Check sheet for the modelled part. Datum: model origin and axes. Units: mm. A direction names the side the tool comes from. Round coordinates to 2 decimals unless told otherwise and drop trailing zeros. Order: outer loops, then holes, each group sorted by start corner. A loop starts at its lowest first (then second) coordinate and runs counter-clockwise, first axis right, second up. Notation, with made-up numbers: (34, 12.25) -> (49, 12.25) arc R22 cw to (49, 27.25) -> close; hole circle Ø10 at (-14.75, -5.75). An arc over 180 degrees is marked (long way). Answer in a Markdown table with one row per item.
from build123d import *

# Parameters (mm, degrees)
SKETCH1_R                                       = 12
SKETCH1_R_2                                     = 1.65
BOSS_EXTRUDE1_DEPTH                             = 15
SKETCH2_R                                       = 20
SKETCH2_R_2                                     = 11.285963192
BOSS_EXTRUDE2_DEPTH                             = 5
SKETCH3_R                                       = 20
BOSS_EXTRUDE3_DEPTH                             = 3
CUT_EXTRUDE2_DEPTH                              = 2.1
SKETCH6_R                                       = 1.65
CUT_EXTRUDE3_DEPTH                              = 24.1
FILLET1_R                                       = 1
SKETCH7_R                                       = 3.5
CUT_EXTRUDE4_DEPTH                              = 5.5
CSK_FOR_M3_FLAT_HEAD_MACHINE_SCREW1_D           = 3.4
CSK_FOR_M3_FLAT_HEAD_MACHINE_SCREW1_CSINK_D     = 6.3
CSK_FOR_M3_FLAT_HEAD_MACHINE_SCREW1_CSINK_ANGLE = 90
CUT_EXTRUDE6_DEPTH                              = 2
CUT_EXTRUDE6_DEPTH_BACK                         = 10


with BuildPart() as part:
    # Sketch1 → Boss-Extrude1 (new body)
    with BuildSketch(Plane(origin=(0, 0, 0), x_dir=(1, 0, 0), z_dir=(0, 1, 0))):
        Circle(SKETCH1_R)
        with Locations((0, 7)):
            Circle(SKETCH1_R_2, mode=Mode.SUBTRACT)
        with Locations((7, 0)):
            Circle(SKETCH1_R_2, mode=Mode.SUBTRACT)
        Circle(SKETCH1_R_2, mode=Mode.SUBTRACT)
        with Locations((0, -7)):
            Circle(SKETCH1_R_2, mode=Mode.SUBTRACT)
        with Locations((-7, 0)):
            Circle(SKETCH1_R_2, mode=Mode.SUBTRACT)
    extrude(amount=BOSS_EXTRUDE1_DEPTH)

    # Sketch2 → Boss-Extrude2 (add)
    with BuildSketch(Plane(origin=(0, 15, 0), x_dir=(1, 0, 0), z_dir=(0, 1, 0))):
        Circle(SKETCH2_R)
        Circle(SKETCH2_R_2, mode=Mode.SUBTRACT)
    extrude(amount=-BOSS_EXTRUDE2_DEPTH)

    # Sketch3 → Boss-Extrude3 (add)
    with BuildSketch(Plane(origin=(0, 15, 0), x_dir=(1, 0, 0), z_dir=(0, 1, 0))):
        Circle(SKETCH3_R)
    extrude(amount=-BOSS_EXTRUDE3_DEPTH)

    # Sketch4 → Cut-Extrude2 (cut)
    with BuildSketch(Plane.XZ.offset(-15)):
        with BuildLine():
            Line((4.949747468, 4.949747468), (1.940261042, 16.98516707))
            ThreePointArc((1.940261042, 16.98516707), (0, 18.5), (-1.940261043, 16.98516707))
            Line((-1.940261043, 16.98516707), (-4.949747468, 4.949747468))
            Line((-4.949747468, 4.949747468), (-16.98516707, 1.940261042))
            ThreePointArc((-16.98516707, 1.940261042), (-18.5, 0), (-16.98516707, -1.940261043))
            Line((-16.98516707, -1.940261043), (-4.949747468, -4.949747468))
            Line((-4.949747468, -4.949747468), (-1.940261042, -16.98516707))
            ThreePointArc((-1.940261042, -16.98516707), (0, -18.5), (1.940261043, -16.98516707))
            Line((1.940261043, -16.98516707), (4.949747468, -4.949747468))
            Line((4.949747468, -4.949747468), (16.98516707, -1.940261042))
            ThreePointArc((16.98516707, -1.940261042), (18.5, 0), (16.98516707, 1.940261043))
            Line((16.98516707, 1.940261043), (4.949747468, 4.949747468))
        make_face()
    extrude(amount=CUT_EXTRUDE2_DEPTH, mode=Mode.SUBTRACT)

    # Sketch6 → Cut-Extrude3 (cut)
    with BuildSketch(Plane.XZ):
        Circle(SKETCH6_R)
    extrude(amount=-CUT_EXTRUDE3_DEPTH, mode=Mode.SUBTRACT)

    # Fillet1
    fillet1_edges = [part.edges().sort_by_distance(p)[0] for p in [
        (4.949747468, 13.95, 4.949747468),
        (-4.949747468, 13.95, 4.949747468),
        (-4.949747468, 13.95, -4.949747468),
        (4.949747468, 13.95, -4.949747468),
    ]]
    fillet(fillet1_edges, radius=FILLET1_R)

    # Sketch7 → Cut-Extrude4 (cut)
    with BuildSketch(Plane.XZ):
        Circle(SKETCH7_R)
    extrude(amount=-CUT_EXTRUDE4_DEPTH, mode=Mode.SUBTRACT)

    # CSK for M3 Flat Head Machine Screw1 (through all)
    with Locations(Plane(origin=(0, 5.5, 0), x_dir=(-1, 0, 0), z_dir=(0, -1, 0))):
        with Locations((0, 0)):
            CounterSinkHole(CSK_FOR_M3_FLAT_HEAD_MACHINE_SCREW1_D / 2, CSK_FOR_M3_FLAT_HEAD_MACHINE_SCREW1_CSINK_D / 2, counter_sink_angle=CSK_FOR_M3_FLAT_HEAD_MACHINE_SCREW1_CSINK_ANGLE)

    # Sketch12 → Cut-Extrude6 (cut, two sides)
    with BuildSketch(Plane.XZ.offset(-12)) as cut_extrude6_sk:
        with BuildLine():
            Line((-2.836233197, 8.522029946), (-2.836233197, 5.477970054))
            ThreePointArc((-2.836233197, 5.477970054), (-2.809438278, 5.377970054), (-2.736233197, 5.304764973))
            Line((-2.736233197, 5.304764973), (-0.1, 3.782735027))
            ThreePointArc((-0.1, 3.782735027), (0, 3.755940108), (0.1, 3.782735027))
            Line((0.1, 3.782735027), (2.736233197, 5.304764973))
            ThreePointArc((2.736233197, 5.304764973), (2.809438278, 5.377970054), (2.836233197, 5.477970054))
            Line((2.836233197, 5.477970054), (2.836233197, 8.522029946))
            ThreePointArc((2.836233197, 8.522029946), (2.809438278, 8.622029946), (2.736233197, 8.695235027))
            Line((2.736233197, 8.695235027), (0.1, 10.217264973))
            ThreePointArc((0.1, 10.217264973), (0, 10.244059892), (-0.1, 10.217264973))
            Line((-0.1, 10.217264973), (-2.736233197, 8.695235027))
            ThreePointArc((-2.736233197, 8.695235027), (-2.809438278, 8.622029946), (-2.836233197, 8.522029946))
        make_face()
        with BuildLine():
            Line((-10.217264973, -0.1), (-8.695235027, -2.736233197))
            ThreePointArc((-8.695235027, -2.736233197), (-8.622029946, -2.809438278), (-8.522029946, -2.836233197))
            Line((-8.522029946, -2.836233197), (-5.477970054, -2.836233197))
            ThreePointArc((-5.477970054, -2.836233197), (-5.377970054, -2.809438278), (-5.304764973, -2.736233197))
            Line((-5.304764973, -2.736233197), (-3.782735027, -0.1))
            ThreePointArc((-3.782735027, -0.1), (-3.755940108, 0), (-3.782735027, 0.1))
            Line((-3.782735027, 0.1), (-5.304764973, 2.736233197))
            ThreePointArc((-5.304764973, 2.736233197), (-5.377970054, 2.809438278), (-5.477970054, 2.836233197))
            Line((-5.477970054, 2.836233197), (-8.522029946, 2.836233197))
            ThreePointArc((-8.522029946, 2.836233197), (-8.622029946, 2.809438278), (-8.695235027, 2.736233197))
            Line((-8.695235027, 2.736233197), (-10.217264973, 0.1))
            ThreePointArc((-10.217264973, 0.1), (-10.244059892, 0), (-10.217264973, -0.1))
        make_face()
        with BuildLine():
            Line((8.522029946, 2.836233197), (5.477970054, 2.836233197))
            ThreePointArc((5.477970054, 2.836233197), (5.377970054, 2.809438278), (5.304764973, 2.736233197))
            Line((5.304764973, 2.736233197), (3.782735027, 0.1))
            ThreePointArc((3.782735027, 0.1), (3.755940108, 0), (3.782735027, -0.1))
            Line((3.782735027, -0.1), (5.304764973, -2.736233197))
            ThreePointArc((5.304764973, -2.736233197), (5.377970054, -2.809438278), (5.477970054, -2.836233197))
            Line((5.477970054, -2.836233197), (8.522029946, -2.836233197))
            ThreePointArc((8.522029946, -2.836233197), (8.622029946, -2.809438278), (8.695235027, -2.736233197))
            Line((8.695235027, -2.736233197), (10.217264973, -0.1))
            ThreePointArc((10.217264973, -0.1), (10.244059892, 0), (10.217264973, 0.1))
            Line((10.217264973, 0.1), (8.695235027, 2.736233197))
            ThreePointArc((8.695235027, 2.736233197), (8.622029946, 2.809438278), (8.522029946, 2.836233197))
        make_face()
        with BuildLine():
            Line((2.836233197, -8.522029946), (2.836233197, -5.477970054))
            ThreePointArc((2.836233197, -5.477970054), (2.809438278, -5.377970054), (2.736233197, -5.304764973))
            Line((2.736233197, -5.304764973), (0.1, -3.782735027))
            ThreePointArc((0.1, -3.782735027), (0, -3.755940108), (-0.1, -3.782735027))
            Line((-0.1, -3.782735027), (-2.736233197, -5.304764973))
            ThreePointArc((-2.736233197, -5.304764973), (-2.809438278, -5.377970054), (-2.836233197, -5.477970054))
            Line((-2.836233197, -5.477970054), (-2.836233197, -8.522029946))
            ThreePointArc((-2.836233197, -8.522029946), (-2.809438278, -8.622029946), (-2.736233197, -8.695235027))
            Line((-2.736233197, -8.695235027), (-0.1, -10.217264973))
            ThreePointArc((-0.1, -10.217264973), (0, -10.244059892), (0.1, -10.217264973))
            Line((0.1, -10.217264973), (2.736233197, -8.695235027))
            ThreePointArc((2.736233197, -8.695235027), (2.809438278, -8.622029946), (2.836233197, -8.522029946))
        make_face()
    extrude(amount=CUT_EXTRUDE6_DEPTH, mode=Mode.SUBTRACT)
    extrude(cut_extrude6_sk.sketch, amount=-CUT_EXTRUDE6_DEPTH_BACK, mode=Mode.SUBTRACT)


solid = part.part
Item 1: Cross-section at D-D (x = -15). Record the boundary of the cut face in (y, z), and give its area (3 significant figures).
Result sheet:
| item | result |
|---|---|
| outline | (10, -13.23) -> (15, -13.23) -> (15, -2.44) -> (12.9, -2.44) -> (12.9, 2.44) -> (15, 2.44) -> (15, 13.23) -> (10, 13.23) -> close |
| area | 122 mm^2 |
Item 2: Depth check by flat-ended pin: P1, Ø4.5, axis at x = -7.5, z = -1, coming from the +Y side; P2, Ø7.5, axis at x = 0.5, z = 1, coming from the -Y side; P3, Ø1.5, axis at x = -6.5, y = 11.5, coming from the -Z side; P4, Ø1.5, axis at x = 7.5, y = 11, coming from the -Z side. Enter the tip coordinate at first touch or a pass-through.
Result sheet:
| item | result |
|---|---|
| P1 | stops at y = 12.9 |
| P2 | stops at y = 0 |
| P3 | stops at z = -19.16 |
| P4 | stops at z = -18.83 |
Item 3: Cross-section at B-B (z = -7). Record the boundary of the cut face in (x, y) (3 decimals).
Result sheet:
| item | result |
|---|---|
| outline | (-18.735, 10) -> (-9.747, 10) -> (-9.747, 0) -> (-1.65, 0) -> (-1.65, 10) -> (-2.836, 10) -> (-2.836, 12.9) -> (-4.437, 12.9) -> (-4.437, 15) -> (-18.735, 15) -> close; (1.65, 0) -> (9.747, 0) -> (9.747, 10) -> (18.735, 10) -> (18.735, 15) -> (4.437, 15) -> (4.437, 12.9) -> (2.836, 12.9) -> (2.836, 10) -> (1.65, 10) -> close |
Item 4: Cross-section at C-C (x = -7). Record the boundary of the cut face in (y, z) (3 decimals), and give its area (3 significant figures).
Result sheet:
| item | result |
|---|---|
| outline | (0, -9.747) -> (10, -9.747) -> (10, -18.735) -> (15, -18.735) -> (15, -4.437) -> (12.9, -4.437) -> (12.9, -2.836) -> (10, -2.836) -> (10, -1.65) -> (0, -1.65) -> close; (0, 1.65) -> (10, 1.65) -> (10, 2.836) -> (12.9, 2.836) -> (12.9, 4.437) -> (15, 4.437) -> (15, 18.735) -> (10, 18.735) -> (10, 9.747) -> (0, 9.747) -> close |
| area | 314 mm^2 |
Item 5: Mould release check, pull along X, two halves, no side actions. Record for faces 1 (the flat face through (-4.533, 11.43, 1.4)), 2 (the flat face through (9, 10, 9)): pulls with the +X half, pulls with the -X half, needs draft (parallel to the pull), parting line crosses it, or undercut.
Result sheet:
| item | result |
|---|---|
| face 1 | undercut |
| face 2 | needs draft |
Item 6: Set-up check for faces 3 (the cylindrical face through (-8.65, 4.93, -0.07)), 4 (the flat face through (1.2, 10, -8.4)): record each of +Z, -Z, +X, -X, +Y, -Y from which the full face is reachable in a straight line by a thin tool's end or side.
Result sheet:
| item | result |
|---|---|
| face 3 | +Y, -Y |
| face 4 | +Y |
Item 7: Scan lines: line 1 (Z direction, x = 0, y = 10.75); line 2 (Z direction, x = 0.5, y = 6.75); line 3 (Y direction, x = -12.5, z = 15). Record each from-to range of solid material in increasing order. Write a range as [from, to].
Result sheet:
| item | result |
|---|---|
| line 1 | z = [-20, -10.24], [-3.76, -1.7], [1.7, 3.76], [10.24, 20] |
| line 2 | z = [-11.99, -8.57], [-5.43, -1.83], [1.83, 5.43], [8.57, 11.99] |
| line 3 | y = [10, 15] |
Item 8: Cross-section at A-A (y = 8.5). Record the boundary of the cut face in (x, z), and give its area (3 significant figures).
Result sheet:
| item | result |
|---|---|
| outline | circle Ø24 at (0, 0); hole circle Ø3.3 at (-7, 0); hole circle Ø3.4 at (0, 0); hole circle Ø3.3 at (0, -7); hole circle Ø3.3 at (0, 7); hole circle Ø3.3 at (7, 0) |
| area | 409 mm^2 |
